```python
from build123d import *

# Parameters (mm, degrees)
BOSS_EXTRUDE1_DEPTH = 25
CUT_EXTRUDE2_DEPTH  = 26
BOSS_EXTRUDE2_DEPTH = 0.4


with BuildPart() as part:
    # Sketch1 → Boss-Extrude1 (new body)
    with BuildSketch(Plane(origin=(0, 0, 0), x_dir=(1, 0, 0), z_dir=(0, 1, 0))):
        with BuildLine():
            ThreePointArc((1.451818925, -34.068556857), (1.641248992, -34.346908706), (1.964225605, -34.442038138))
            ThreePointArc((1.964225605, -34.442038138), (26.591847487, -21.978073076), (34.198225299, 4.555174015))
            ThreePointArc((34.198225299, 4.555174015), (23.590291339, 25.176355888), (2.324135821, 34.423627607))
            ThreePointArc((2.324135821, 34.423627607), (1.751838249, 34.289058819), (1.354061739, 33.856153382))
            ThreePointArc((1.354061739, 33.856153382), (0, 33.001534515), (-1.354061739, 33.856153382))
            ThreePointArc((-1.354061739, 33.856153382), (-1.751838249, 34.289058819), (-2.324135821, 34.423627607))
            ThreePointArc((-2.324135821, 34.423627607), (-23.590291339, 25.176355888), (-34.198225299, 4.555174015))
            ThreePointArc((-34.198225299, 4.555174015), (-26.591847487, -21.978073076), (-1.964225605, -34.442038138))
            ThreePointArc((-1.964225605, -34.442038138), (-1.641248992, -34.346908706), (-1.451818925, -34.068556857))
            ThreePointArc((-1.451818925, -34.068556857), (0, -32.945679925), (1.451818925, -34.068556857))
        make_face()
        with BuildLine():
            Line((-2.417, 3.787737139), (0, 3.787737139))
            Line((0, 3.787737139), (2.417, 3.787737139))
            ThreePointArc((2.417, 3.787737139), (0, -4.489512172), (-2.417, 3.787737139))
        make_face(mode=Mode.SUBTRACT)
    extrude(amount=BOSS_EXTRUDE1_DEPTH)

    # Sketch2 → Cut-Extrude2 (cut, through all)
    with BuildSketch(Plane(origin=(0, 0, 0), x_dir=(1, 0, 0), z_dir=(0, 1, 0))):
        with BuildLine():
            ThreePointArc((-31.360169492, -2.964754537), (-22.273863607, -22.273863607), (-2.964754537, -31.360169492))
            ThreePointArc((-2.964754537, -31.360169492), (-1.977522645, -31.202516837), (-1.189935494, -30.586734694))
            ThreePointArc((-1.189935494, -30.586734694), (0, -30), (1.189935494, -30.586734694))
            ThreePointArc((1.189935494, -30.586734694), (1.977522645, -31.202516837), (2.964754537, -31.360169492))
            ThreePointArc((2.964754537, -31.360169492), (22.273863607, -22.273863607), (31.360169492, -2.964754537))
            ThreePointArc((31.360169492, -2.964754537), (31.202516837, -1.977522645), (30.586734694, -1.189935494))
            ThreePointArc((30.586734694, -1.189935494), (30, 0), (30.586734694, 1.189935494))
            ThreePointArc((30.586734694, 1.189935494), (31.202516837, 1.977522645), (31.360169492, 2.964754537))
            ThreePointArc((31.360169492, 2.964754537), (22.273863607, 22.273863607), (2.964754537, 31.360169492))
            ThreePointArc((2.964754537, 31.360169492), (1.977522645, 31.202516837), (1.189935494, 30.586734694))
            ThreePointArc((1.189935494, 30.586734694), (0, 30), (-1.189935494, 30.586734694))
            ThreePointArc((-1.189935494, 30.586734694), (-1.977522645, 31.202516837), (-2.964754537, 31.360169492))
            ThreePointArc((-2.964754537, 31.360169492), (-22.273863607, 22.273863607), (-31.360169492, 2.964754537))
            ThreePointArc((-31.360169492, 2.964754537), (-31.202516837, 1.977522645), (-30.586734694, 1.189935494))
            ThreePointArc((-30.586734694, 1.189935494), (-30, 0), (-30.586734694, -1.189935494))
            ThreePointArc((-30.586734694, -1.189935494), (-31.202516837, -1.977522645), (-31.360169492, -2.964754537))
        make_face()
    extrude(amount=CUT_EXTRUDE2_DEPTH, mode=Mode.SUBTRACT)

    # Sketch2<2> → Boss-Extrude2 (add)
    with BuildSketch(Plane(origin=(0, 0, 0), x_dir=(1, 0, 0), z_dir=(0, 1, 0))):
        with BuildLine():
            ThreePointArc((-31.360169492, -2.964754537), (-22.273863607, -22.273863607), (-2.964754537, -31.360169492))
            ThreePointArc((-2.964754537, -31.360169492), (-1.977522645, -31.202516837), (-1.189935494, -30.586734694))
            ThreePointArc((-1.189935494, -30.586734694), (0, -30), (1.189935494, -30.586734694))
            ThreePointArc((1.189935494, -30.586734694), (1.977522645, -31.202516837), (2.964754537, -31.360169492))
            ThreePointArc((2.964754537, -31.360169492), (22.273863607, -22.273863607), (31.360169492, -2.964754537))
            ThreePointArc((31.360169492, -2.964754537), (31.202516837, -1.977522645), (30.586734694, -1.189935494))
            ThreePointArc((30.586734694, -1.189935494), (30, 0), (30.586734694, 1.189935494))
            ThreePointArc((30.586734694, 1.189935494), (31.202516837, 1.977522645), (31.360169492, 2.964754537))
            ThreePointArc((31.360169492, 2.964754537), (22.273863607, 22.273863607), (2.964754537, 31.360169492))
            ThreePointArc((2.964754537, 31.360169492), (1.977522645, 31.202516837), (1.189935494, 30.586734694))
            ThreePointArc((1.189935494, 30.586734694), (0, 30), (-1.189935494, 30.586734694))
            ThreePointArc((-1.189935494, 30.586734694), (-1.977522645, 31.202516837), (-2.964754537, 31.360169492))
            ThreePointArc((-2.964754537, 31.360169492), (-22.273863607, 22.273863607), (-31.360169492, 2.964754537))
            ThreePointArc((-31.360169492, 2.964754537), (-31.202516837, 1.977522645), (-30.586734694, 1.189935494))
            ThreePointArc((-30.586734694, 1.189935494), (-30, 0), (-30.586734694, -1.189935494))
            ThreePointArc((-30.586734694, -1.189935494), (-31.202516837, -1.977522645), (-31.360169492, -2.964754537))
        make_face()
    extrude(amount=BOSS_EXTRUDE2_DEPTH)


solid = part.part
```
For this review, take the finished solid that the model builds, in its own axes (mm). A direction names the side the tool comes from. Round coordinates to 2 decimals unless told otherwise and drop trailing zeros. Write each loop counter-clockwise with the first axis right and the second up, starting at its lowest first coordinate (ties: lowest second). Pieces come first, ordered by that corner, then holes. Notation, with made-up numbers: (-16, -24.5) - (-1, -24.5) arc R23 cw to (-1, 4.5) - close; hole circle Ø8 at (-16, -27.75). An arc over 180 degrees is marked (long way). Write each question's results on one line, items separated by ' | '.
Item 1: Draft analysis for pull direction X (two halves, no side actions). For faces 3 (the face through (-0.2, 25, 30.5)), 4 (the face through (31.21, 12.53, 1.99)), state which applies: pulls with the +X half, pulls with the -X half, needs draft (parallel to the pull), parting line crosses it, or undercut.
Calculated:
face 3: needs draft | face 4: undercut
Item 2: Take a section at B-B on z = 5. State the section outline as (x, y) points, then the cut area to 3 significant figures.
Calculated:
outline: (-34.14, 0) - (34.14, 0) - (34.14, 25) - (31.1, 25) - (31.1, 0.4) - (-31.1, 0.4) - (-31.1, 25) - (-34.14, 25) - close | area: 177 mm^2
Item 3: To check wall thickness, follow line 1 along X through (y, z) = (10.5, 0); line 2 along Y through (x, z) = (-22, 22); line 3 along Z through (x, y) = (11, 23.25). State the ranges of each line that lie inside material, in increasing order. Write a range as from..to.
Calculated:
line 1: x = -34.5..-30, 30..34.5 | line 2: y = 0..0.4 | line 3: z = -32.7..-29.52, 29.52..32.7
Item 4: For faces 1 (the face through (0, 0, 0)), 2 (the face through (1.99, 12.53, -31.21)), list the 3-axis set-ups (+Z, -Z, +X, -X, +Y, -Y) from which the entire face can be reached by the end or side of a thin tool; tool diameter is ignored.
Calculated:
face 1: +Z, -Z, +X, -X, -Y | face 2: +Y
Item 5: For pin 1 (1 mm diameter, centred on x = 9, z = -5.5, fed in from -Y); pin 2 (10 mm diameter, centred on x = 12, y = 16, fed in from -Z); pin 3 (2 mm diameter, centred on x = -25.5, y = 16, fed in from +Z); pin 4 (5 mm diameter, centred on x = -23, y = 18.5, fed in from -Z), all flat-tipped, find the tip position at first contact; note any pin that passes through.
Calculated:
pin 1: stops at y = 0 | pin 2: stops at z = -33.78 | pin 3: stops at z = 24.29 | pin 4: stops at z = -27.75
Item 6: Take a section at C-C on x = 24.5. State the section outline as (y, z) points.
Calculated:
outline: (0, -24.29) - (25, -24.29) - (25, -19.8) - (0.4, -19.8) - (0.4, 19.8) - (25, 19.8) - (25, 24.29) - (0, 24.29) - close
